Here's how the part is built. I have some questions about the finished solid (model axes, mm). A direction names the side the tool comes from. Coordinates: 2 decimals unless noted, no trailing zeros. Write each loop counter-clockwise with the first axis right and the second up, starting at its lowest first coordinate (ties: lowest second). Pieces come first, ordered by that corner, then holes.
from build123d import *

# Parameters (mm, degrees)
SKETCH_4_W          = 114
SKETCH_4_H          = 138
EXTRUDE_1_DEPTH     = 59
SHELL_1_T           = -1
SKETCH_5_W          = 114
SKETCH_5_H          = 12
EXTRUDE_2_DEPTH     = 11
SKETCH_6_W          = 112
SKETCH_6_H          = 10
CUT_EXTRUDE_1_DEPTH = 11


with BuildPart() as part:
    # 草图4 → 凸台-拉伸1 (new body)
    with BuildSketch(Plane(origin=(0, 0, 0), x_dir=(1, 0, 0), z_dir=(0, 1, 0))):
        Rectangle(SKETCH_4_W, SKETCH_4_H)
    extrude(amount=EXTRUDE_1_DEPTH)

    # 抽壳1
    shell_1_openings = [part.faces().sort_by_distance(p)[0] for p in [
        (0, 59, 0),
    ]]
    offset(amount=SHELL_1_T, openings=shell_1_openings, kind=Kind.INTERSECTION)

    # 草图5 → 凸台-拉伸2 (add)
    with BuildSketch(Plane.XY.offset(69)):
        with Locations((0, 53)):
            Rectangle(SKETCH_5_W, SKETCH_5_H)
    extrude(amount=EXTRUDE_2_DEPTH)

    # 草图6 → 切除-拉伸1 (cut)
    with BuildSketch(Plane.XZ.offset(-47)):
        with Locations((0, 74)):
            Rectangle(SKETCH_6_W, SKETCH_6_H)
    extrude(amount=-CUT_EXTRUDE_1_DEPTH, mode=Mode.SUBTRACT)


solid = part.part
1. I want a section at A-A (y = 49.5). List the corners of the cut face in (x, z) for me.
2. I want a section at D-D (x = -23.5). List the corners of the cut face in (y, z) for me, then the cut area to 3 significant figures.
3. I want a section at B-B (y = 23.5). List the corners of the cut face in (x, z) for me, then the cut area to 3 significant figures.
4. Thinking about a two-plate mould opening in X: for faces 5 (the face through (-1, 29, 69)), 6 (the face through (57, 29, 4)), 7 (the face through (-1, 1, -1)), 8 (the face through (-1, 29, -69)), which applies, pulls with the +X half, pulls with the -X half, needs draft (parallel to the pull), parting line crosses it, or undercut?
5. If I drill on line 1 (Z direction, x = 23, y = 54.5); line 2 (X direction, y = 22.5, z = -54); line 3 (Z direction, x = -10, y = 38), over which ranges is the centre line in solid material (lowest first)?
6. For pin 1 Ø12 at (x, z) = (-9.5, 75.5) entering from -Y; pin 2 Ø5 at (x, z) = (18, 74) entering from -Y, each with a flat end and sliding along its axis, tell me the tip position at first contact or that it passes through.
7. I want a section at C-C (z = -14). List the corners of the cut face in (x, y) for me, then the cut area to 3 significant figures.
8. On a 3-axis mill with a long thin cutter (end or side, diameter ignored), from which of +Z, -Z, +X, -X, +Y, -Y can I reach the whole of each face in a straight line? I mean faces 1 (the face through (-1, 52, 79)), 2 (the face through (-0.3, 47, 79.4)), 3 (the face through (-56, 30, 1)), 4 (the face through (-1, 53, 80)). Say none if no direction works.
Response values:
1. outline: (-57, -69) - (57, -69) - (57, 80) - (-57, 80) - close; hole (-56, -68) - (56, -68) - (56, 68) - (-56, 68) - close; hole (-56, 69) - (56, 69) - (56, 79) - (-56, 79) - close
2. outline: (0, -69) - (59, -69) - (59, -68) - (1, -68) - (1, 68) - (59, 68) - (59, 80) - (47, 80) - (47, 79) - (58, 79) - (58, 69) - (0, 69) - close
2. area: 276 mm2
3. outline: (-57, -69) - (57, -69) - (57, 69) - (-57, 69) - close; hole (-56, -68) - (56, -68) - (56, 68) - (-56, 68) - close
3. area: 500 mm2
4. face 5: undercut
4. face 6: pulls with the +X half
4. face 7: undercut
4. face 8: needs draft
5. line 1: z = -69 to -68, 68 to 69, 79 to 80
5. line 2: x = -57 to -56, 56 to 57
5. line 3: z = -69 to -68, 68 to 69
6. pin 1: stops at y = 47
6. pin 2: stops at y = 58
7. outline: (-57, 0) - (57, 0) - (57, 59) - (56, 59) - (56, 1) - (-56, 1) - (-56, 59) - (-57, 59) - close
7. area: 230 mm2
8. face 1: -Y
8. face 2: +Z, +X, -X, -Y
8. face 3: +Y
8. face 4: +Z, +X, -X, +Y, -Y
